Autodesk Inventor part; units mm, degrees
ref_plane "YZ Plane" through (0, 0, 0) normal (1, 0, 0) x (0, 1, 0)
ref_plane "XZ Plane" through (0, 0, 0) normal (0, 1, 0) x (-1, 0, 0)
ref_plane "XY Plane" through (0, 0, 0) normal (0, 0, 1) x (1, 0, 0)
sketch "Sketch1" plane through (0, 0, 0) normal (0, 1, 0) x (-1, 0, 0)
  line L0 (0, 0) -> (0, -50.8)
  line L1 (0, -50.8) -> (76.2, -127)
  line L2 (127, -127) -> (76.2, -127)
  line L3 (0, 0) -> (127, 0)
  line L4 (127, 0) -> (533.4, 0)
  line L5 (533.4, 0) -> (533.4, -127)
  line L6 (533.4, -127) -> (127, -127)
  dimension "d7" = 135
  dimension "d37" = 406.4
extrude "Extrusion1" add sketch "Sketch1" along normal blind 127
sketch "Sketch2" plane through (-76.2, 0, -127) normal (0.7071, 0, -0.7071) x (-0.7071, 0, -0.7071)
  line L0 (-107.7631, 0) -> (0, 0)
  line L1 (0, 0) -> (0, 127)
  line L2 (-107.7631, 127) -> (0, 127)
  line L3 (-107.7631, 0) -> (-107.7631, 127)
  line L4 (-107.7631, -190.5) -> (0.0091, -190.5)
  line L5 (0.0091, -190.5) -> (0.0091, 317.5)
  line L6 (0.0091, 317.5) -> (-107.7631, 317.5)
  line L7 (-107.7631, -190.5) -> (-107.7631, 317.5)
  point P0 (-143.6841, 0)
  dimension "d9" = 107.7722
  dimension "d10" = 508
extrude "Extrusion2" add sketch "Sketch2" along normal blind 101.6
sketch "Sketch3" plane through (-76.2065, -190.5, -127.0065) normal (-0.7071, 0, -0.7071) x (-0.7071, 0, 0.7071)
  line L0 (0, 0) -> (-101.6, 0)
  line L1 (0, 508) -> (-101.6, 508)
  circle A0 centre (-50.8, 50.8) radius 44.45
  circle A1 centre (-50.8, 152.4) radius 44.45
  circle A2 centre (-50.8, 254) radius 44.45
  circle A3 centre (-50.8, 355.6) radius 44.45
  circle A4 centre (-50.8, 457.2) radius 44.45
  point P0 (35.921, 190.5)
extrude "Extrusion3" cut sketch "Sketch3" against normal blind 127
sketch "Sketch4" plane through (-533.4, 0, -127) normal (-1, 0, 0) x (0, 0, 1)
  line L0 (0, 0) -> (0, 127) construction
  line L1 (76.2, 0) -> (0, 0) construction
  line L2 (0, 63.5) -> (76.2, 0) construction
  line L3 (76.2, 0) -> (127, 63.5) construction
  line L4 (127, 0) -> (127, 127) construction
  line L5 (76.2, 127) -> (0, 127) construction
  line L6 (0, 63.5) -> (76.2, 127) construction
  line L7 (76.2, 127) -> (127, 63.5) construction
  line L8 (38.1, 31.75) -> (101.6, 31.75) construction
  line L9 (38.1, 95.25) -> (101.6, 95.25) construction
  circle A0 centre (38.1, 31.75) radius 6.35
  circle A1 centre (38.1, 95.25) radius 6.35
  circle A2 centre (101.6, 95.25) radius 6.35
  circle A3 centre (101.6, 31.75) radius 6.35
  dimension "d38" = 12.7
  dimension "d39" = 12.7
  dimension "d40" = 12.7
  dimension "d41" = 12.7
extrude "Extrusion4" add sketch "Sketch4" along normal blind 25.4
thread "Thread1"
thread "Thread2"
thread "Thread3"
thread "Thread4"
properties part number "TubeHolderV3"
Geometry check sheet. Reference: the model listing, model coordinates, mm. A direction names the side the tool comes from. Round coordinates to 2 decimals unless told otherwise and drop trailing zeros. Order: outer loops, then holes, each group sorted by start corner. A loop starts at its lowest first (then second) coordinate and runs counter-clockwise, first axis right, second up. Notation, with made-up numbers: M -9,-1.5 L 38,-1.5 A19 ccw 38,4.5 Z; hole C 59,71 d4. An arc over 180 degrees is marked long. Write item = value, one per line.
Q1. Section check B-B (x = -358.5). Enter the section's corners in (y, z).
Answer block:
outline = M 0,-127 L 127,-127 L 127,0 L 0,0 Z
Q2. Section check C-C (y = -146.5). Enter the section's corners in (x, z), plus the area to 3 significant figures.
Answer block:
outline = M -76.21,-127.01 L -71.35,-131.87 L 4.86,-55.66 L 0,-50.8 Z; M -9.22,-193.99 L -4.36,-198.85 L 71.84,-122.64 L 66.98,-117.78 Z
area = 1,480 mm^2
Q3. Section check A-A (y = -67). Enter the section's corners in (x, z).
Answer block:
outline = M -76.21,-127.01 L -64.17,-139.05 L 12.04,-62.84 L 0,-50.8 Z; M -16.4,-186.81 L -4.36,-198.85 L 71.84,-122.64 L 59.8,-110.6 Z
Q4. Release check for a two-part mould opening along Z. For faces 1 (the flat face through (-558.8, 95, -89)), 2 (the cylindrical face through (1.38, 107.57, -129.45)), 3 (the flat face through (-37.6, -45.8, -88.4)) record: released by +Z, released by -Z, zero draft, split by the parting line, or undercut.
Answer block:
face_1 = zero draft
face_2 = undercut
face_3 = released by +Z
Q5. Depth check by flat-ended pin: pin 1 Ø15 at (y, z) = (46, -24.5) entering from +X; pin 2 Ø10 at (x, z) = (-366.5, -79.5) entering from -Y. Enter the tip coordinate at first touch or a pass-through.
Answer block:
pin_1 = 0
pin_2 = 0
Q6. Set-up check for faces 4 (the cylindrical face through (-545.92, 101.45, -26.78)), 5 (the flat face through (-308, 63, -127)), 6 (the flat face through (3.5, 59.9, -54.3)): record each of +Z, -Z, +X, -X, +Y, -Y from which the full face is reachable in a straight line by a thin tool's end or side.
Answer block:
face_4 = -X
face_5 = -Z, -X, +Y, -Y
face_6 = +Z, +X, +Y, -Y
Q7. Scan lines: line 1 (X direction, y = 108.5, z = -39); line 2 (Y direction, x = -235.5, z = -112); line 3 (Y direction, x = 28.5, z = -116.5). Record each from-to range of solid material in increasing order.
Answer block:
line_1 = -533.4 to 0
line_2 = 0 to 127
line_3 = -190.5 to -181.24, -98.16 to -79.64, 3.44 to 21.96, 105.04 to 123.56, 206.64 to 225.16, 308.24 to 317.5
